Geometry: final body of the model. Coordinates: model frame, mm. Give positions to 0.01 mm unless a question says otherwise; leave off trailing zeros. Loops run counter-clockwise (first coordinate to the right, second up) from the corner with the lowest first, then second, coordinate; pieces in that order, holes last. Notation, with made-up numbers: (47.25, 84.5) -> (71.25, 84.5) arc R28 ccw to (71.25, 116.5) -> close; hole circle Ø10 at (-22.5, 32). An arc over 180 degrees is marked (long way). One line per item, written item: value. Start each with the question number.
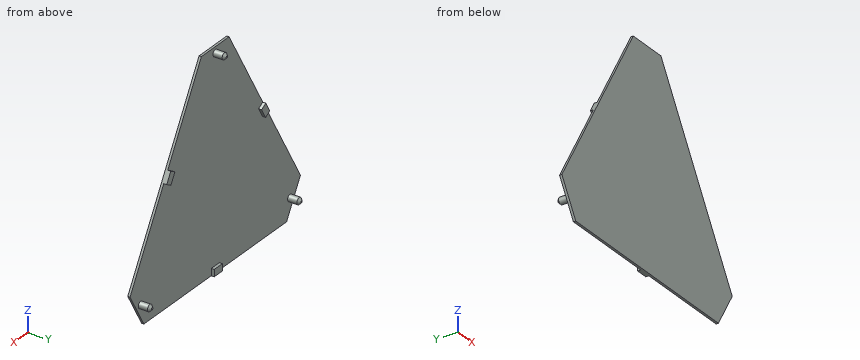
from build123d import *

# Parameters (mm, degrees)
BOSS_EXTRU_2_DEPTH      = 1
ESQUISSE3_R             = 1.45
BOSS_EXTRU_3_DEPTH      = 5
CHANFREIN1_SIZE         = 1
BOSS_EXTRU_4_DEPTH      = 1.3
BOSS_EXTRU_4_DEPTH_BACK = 1
ESQUISSE4_W             = 5
ESQUISSE4_H             = 3


with BuildPart() as part:
    # Esquisse2 → Boss.-Extru.2 (new body)
    with BuildSketch(Plane(origin=(0, 0, 0), x_dir=(1, 0, 0), z_dir=(0, 1, 0))):
        Polygon((-53.339745962, 20.79571669), (-44.679491924, 35.79571669), (44.679491924, 35.79571669), (53.339745962, 20.79571669), (8.660254038, -56.59143338), (-8.660254038, -56.59143338), align=None)
    extrude(amount=BOSS_EXTRU_2_DEPTH)

    # Esquisse3 → Boss.-Extru.3 (add)
    with BuildSketch(Plane(origin=(0, 1, 0), x_dir=(1, 0, 0), z_dir=(0, 1, 0))):
        with Locations(Location((0, -54, 0), (0, 0, 90))):
            Circle(ESQUISSE3_R)
        with Locations(Location((-46.765371804, 27, 0), (0, 0, 90))):
            Circle(ESQUISSE3_R)
        with Locations(Location((46.765371804, 27, 0), (0, 0, 90))):
            Circle(ESQUISSE3_R)
    extrude(amount=BOSS_EXTRU_3_DEPTH)

    # Chanfrein1
    chanfrein1_edges = [part.edges().sort_by_distance(p)[0] for p in [
        (0, 6, 55.45),
        (-46.765371804, 6, -25.55),
        (46.765371804, 6, -25.55),
    ]]
    chamfer(chanfrein1_edges, length=CHANFREIN1_SIZE)

    # Esquisse4 → Boss.-Extru.4 (add, two sides: drawn at the far end of the back side and taken through both)
    with BuildSketch(Plane(origin=(0, 1, 0), x_dir=(1, 0, 0), z_dir=(0, 1, 0)).offset(-BOSS_EXTRU_4_DEPTH_BACK)):
        with Locations((0, 34.29571669)):
            Rectangle(ESQUISSE4_W, ESQUISSE4_H)
        Polygon((32.25, -15.732794835), (29.75, -20.062921854), (27.151923789, -18.562921854), (29.651923789, -14.232794835), align=None)
        Polygon((-29.75, -20.062921854), (-32.25, -15.732794835), (-29.651923789, -14.232794835), (-27.151923789, -18.562921854), align=None)
    extrude(amount=BOSS_EXTRU_4_DEPTH + BOSS_EXTRU_4_DEPTH_BACK)


solid = part.part
Item 1: Section A-A, the plane y = 3.3. Output: boundary loops of the cut face in (x, z).
Item 2: Ray query, line 1 along Z through (x, y) = (-13.5, 0.7); line 2 along Y through (x, z) = (41, -21.5); line 3 along Z through (x, y) = (31, 2.2). Return the intervals inside material, ascending. Write a range as [from, to].
Item 3: Section B-B, the plane x = -6. Output: boundary loops of the cut face in (y, z).
Item 4: Section C-C, the plane z = 8. Output: boundary loops of the cut face in (x, y), then the cut area to 3 significant figures.
Item 5: Pin query (flat end, axial travel): pin 1 (1.5 mm diameter, centred on x = 31, z = 17, fed in from +Y); pin 2 (0.6 mm diameter, centred on y = 2, z = -33.5, fed in from -X); pin 3 (0.6 mm diameter, centred on y = 2, z = -34, fed in from +X). Return the tip coordinate at first contact, or that it passes through.
Geometry check:
1. outline: circle Ø2.9 at (-46.77, -27); circle Ø2.9 at (0, 54); circle Ø2.9 at (46.77, -27)
2. line 1: z = [-35.8, 48.21]
2. line 2: y = [0, 1]
2. line 3: z = [15.01, 17.9]
3. outline: (0, -35.8) -> (1, -35.8) -> (1, 56.59) -> (0, 56.59) -> close
4. outline: (-36.71, 0) -> (36.71, 0) -> (36.71, 1) -> (-36.71, 1) -> close
4. area: 73.4 mm2
5. pin 1: stops at y = 2.3
5. pin 2: stops at x = -2.5
5. pin 3: stops at x = 2.5
